Autodesk Inventor part; units mm, degrees
ref_plane "YZ Plane" through (0, 0, 0) normal (1, 0, 0) x (0, 1, 0)
ref_plane "XZ Plane" through (0, 0, 0) normal (0, 1, 0) x (-1, 0, 0)
ref_plane "XY Plane" through (0, 0, 0) normal (0, 0, 1) x (1, 0, 0)
sketch "Szkic1" plane through (0, 0, 0) normal (0, 1, 0) x (-1, 0, 0)
  line L0 (30.5, 30.5) -> (-30.5, 30.5)
  line L1 (-30.5, 30.5) -> (-30.5, -30.5)
  line L2 (-30.5, -30.5) -> (30.5, -30.5)
  line L3 (30.5, -30.5) -> (30.5, 30.5)
  point P0 (0, 0)
  point P1 (30.5, 0)
  point P2 (0, -30.5)
  dimension "d0" = 61
  dimension "d1" = 61
extrude "Wyciągnięcie proste1" add sketch "Szkic1" along normal blind 1.6
sketch "Szkic2" plane through (0, 1.6, 0) normal (0, 1, 0) x (1, 0, 0)
  circle A0 centre (21.5, -21.5) radius 2.5
  circle A1 centre (-21.5, 21.5) radius 2.5
  line L0 (-30.5, -30.5) -> (30.5, -30.5)
  line L1 (-30.5, 30.5) -> (-30.5, -30.5)
  line L2 (30.5, 30.5) -> (-30.5, 30.5)
  line L3 (30.5, -30.5) -> (30.5, 30.5)
  point P0 (0, 0)
  dimension "d4" = 5
  dimension "d5" = 5
  dimension "d6" = 9
  dimension "d8" = 9
  dimension "d12" = 9
  dimension "d13" = 9
extrude "Wyciągnięcie proste2" cut sketch "Szkic2" against normal up to surface (1.6 mm away) contours A0 | A1
sketch "Szkic3" plane through (0, 0, 0) normal (0, -1, 0) x (1, 0, 0)
  line L0 (-13.9641, -9.4) -> (-38.9641, -9.4)
  line L1 (-38.9641, -9.4) -> (-38.9641, 8.6)
  line L2 (-38.9641, 8.6) -> (-13.9641, 8.6)
  line L3 (-13.9641, 8.6) -> (-13.9641, -9.4)
  line L4 (-30.5, 30.5) -> (30.5, 30.5)
  line L5 (-30.5, -30.5) -> (-30.5, 30.5)
  point P0 (0, 0)
  dimension "d14" = 18
  dimension "d15" = 25
  dimension "d16" = 21.9
  dimension "d17" = 8.4641
extrude "Wyciągnięcie proste3" add sketch "Szkic3" along normal blind 2.5
sketch "Szkic4" plane through (0, 1.6, 0) normal (0, 1, 0) x (1, 0, 0)
  line L0 (-30.5, -12.5) -> (-20.5, -12.5)
  line L1 (-20.5, -12.5) -> (-20.5, -22.5)
  line L2 (-20.5, -22.5) -> (-30.5, -22.5)
  line L3 (-30.5, -22.5) -> (-30.5, -12.5)
  line L4 (-30.5, -30.5) -> (30.5, -30.5)
  line L5 (-30.5, 30.5) -> (-30.5, -30.5)
  point P0 (0, 0)
  dimension "d20" = 10
  dimension "d21" = 10
  dimension "d22" = 8
extrude "Wyciągnięcie proste4" add sketch "Szkic4" along normal blind 4
properties part number "PCB"
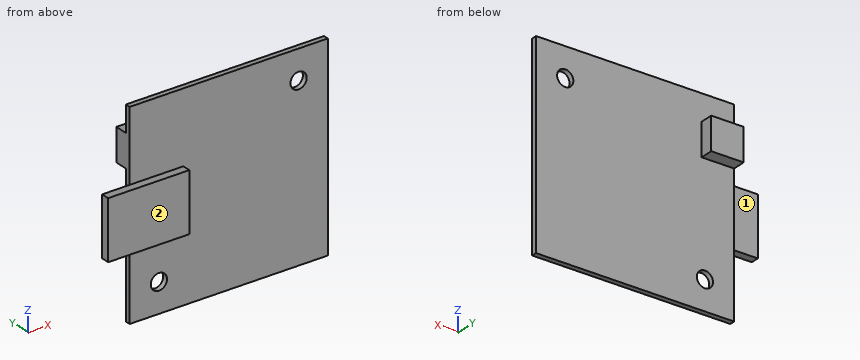
Here's how the part is built. I have some questions about the finished solid (model axes, mm). Face numbers are marked on the shaded views. A direction names the side the tool comes from. Coordinates: 2 decimals unless noted, no trailing zeros. Loops run counter-clockwise (first coordinate to the right, second up) from the corner with the lowest first, then second, coordinate; pieces in that order, holes last. Notation, with made-up numbers: (-11.75, -40) - (38.25, -40) arc R10 ccw to (38.25, -26) - close; hole circle Ø7 at (19.25, 3.25). An arc over 180 degrees is marked (long way). Return JSON: item names as keys, results as strings. Group by question number.
Item 1: On a 3-axis mill with a long thin cutter (end or side, diameter ignored), from which of +Z, -Z, +X, -X, +Y, -Y can I reach the whole of each face in a straight line? I mean the marked faces 1 and 2. Say none if no direction works.
Item 2: I need wall thicknesses on line 1 (X direction, y = 0.9, z = 21.5); line 2 (Z direction, x = -21.5, y = 0.9). Which ranges of each line are inside material? Lowest first, please. Write a range as from..to.
Item 3: If we section it at A-A on z = -21.5: Write out the boundary of the cut face in (x, y).
Item 4: If we section it at B-B on x = -21.5: Write out the boundary of the cut face in (y, z), and give its area (3 significant figures).
Item 5: If we section it at D-D on x = 21.5: Write out the boundary of the cut face in (y, z).
Item 6: Will these pins go through, and if not, where does the flat tip stop? P1, Ø6, axis at x = -17.5, z = -6.5, coming from the +Y side; P2, Ø1.2, axis at y = 3, z = 17, coming from the +X side; P3, Ø3, axis at y = 3, z = 8.5, coming from the -X side.
Item 7: If we section it at C-C on z = 13.5: Write out the boundary of the cut face in (x, y), and give its area (3 significant figures).
Calculated:
{
 "1": {"face 1": "+Z, -Z, -X, +Y", "face 2": "+Z, -Z, +X, -X, -Y"},
 "2": {"line 1": "x = -30.5..19, 24..30.5", "line 2": "z = -30.5..-24, -19..30.5"},
 "3": {"outline": "(-30.5, 0) - (-24, 0) - (-24, 1.6) - (-30.5, 1.6) - close; (-19, 0) - (30.5, 0) - (30.5, 1.6) - (-19, 1.6) - close"},
 "4": {"outline": "(-2.5, -9.4) - (0, -9.4) - (0, -19) - (1.6, -19) - (1.6, 12.5) - (5.6, 12.5) - (5.6, 22.5) - (1.6, 22.5) - (1.6, 30.5) - (0, 30.5) - (0, 8.6) - (-2.5, 8.6) - close; (0, -30.5) - (1.6, -30.5) - (1.6, -24) - (0, -24) - close", "area": "175 mm^2"},
 "5": {"outline": "(0, -30.5) - (1.6, -30.5) - (1.6, 19) - (0, 19) - close; (0, 24) - (1.6, 24) - (1.6, 30.5) - (0, 30.5) - close"},
 "6": {"P1": "stops at y = 1.6", "P2": "stops at x = -20.5", "P3": "stops at x = -30.5"},
 "7": {"outline": "(-30.5, 0) - (30.5, 0) - (30.5, 1.6) - (-20.5, 1.6) - (-20.5, 5.6) - (-30.5, 5.6) - close", "area": "138 mm^2"}
}
